Part model, mm, in its own coordinate system. Round coordinates to 2 decimals unless told otherwise and drop trailing zeros. Order: outer loops, then holes, each group sorted by start corner. A loop starts at its lowest first (then second) coordinate and runs counter-clockwise, first axis right, second up. Notation, with made-up numbers: M -8,27.25 L 41,27.25 A30 cw 41,55.25 Z; hole C 77.5,50 d10. An arc over 180 degrees is marked long. One line per question, with ' | ' between items.
from build123d import *

# Parameters (mm, degrees)
TUBE_SQUARE_40_X_40_X_3_2_1_DEPTH = 1920
CUT_EXTRUDE1_DEPTH                = 1921.52076271
SKETCH16_R                        = 2
CUT_EXTRUDE2_DEPTH                = 3
SKETCH17_R                        = 2
CUT_EXTRUDE3_DEPTH                = 3


with BuildPart() as part:
    # Sketch15 → Tube (square) 40 X 40 X 3.2(1) (new body)
    with BuildSketch(Plane(origin=(0, 0, 0), x_dir=(-1, 0, 0), z_dir=(0, 1, 0))):
        with BuildLine():
            Line((-13.6, -20), (13.6, -20))
            ThreePointArc((13.6, -20), (18.1254834, -18.1254834), (20, -13.6))
            Line((20, -13.6), (20, 13.6))
            ThreePointArc((20, 13.6), (18.1254834, 18.1254834), (13.6, 20))
            Line((13.6, 20), (-13.6, 20))
            ThreePointArc((-13.6, 20), (-18.1254834, 18.1254834), (-20, 13.6))
            Line((-20, 13.6), (-20, -13.6))
            ThreePointArc((-20, -13.6), (-18.1254834, -18.1254834), (-13.6, -20))
        make_face()
        with BuildLine():
            Line((-13.6, -16.8), (13.6, -16.8))
            ThreePointArc((13.6, -16.8), (15.8627417, -15.8627417), (16.8, -13.6))
            Line((16.8, -13.6), (16.8, 13.6))
            ThreePointArc((16.8, 13.6), (15.8627417, 15.8627417), (13.6, 16.8))
            Line((13.6, 16.8), (-13.6, 16.8))
            ThreePointArc((-13.6, 16.8), (-15.8627417, 15.8627417), (-16.8, 13.6))
            Line((-16.8, 13.6), (-16.8, -13.6))
            ThreePointArc((-16.8, -13.6), (-15.8627417, -15.8627417), (-13.6, -16.8))
        make_face(mode=Mode.SUBTRACT)
    extrude(amount=TUBE_SQUARE_40_X_40_X_3_2_1_DEPTH)

    # Sketch13 → Cut-Extrude1 (cut, through all)
    with BuildSketch(Plane(origin=(0, 0, -20), x_dir=(-1, 0, 0), z_dir=(0, 0, -1))):
        Polygon((20, 1880), (-20, 1920), (20, 1920), align=None)
    extrude(amount=-CUT_EXTRUDE1_DEPTH, mode=Mode.SUBTRACT)

    # Sketch16 → Cut-Extrude2 (cut)
    with BuildSketch(Plane(origin=(20, 0, 0), x_dir=(0, 0, -1), z_dir=(1, 0, 0))):
        with Locations((0, 1900)):
            Circle(SKETCH16_R)
        with Locations((0, 1447)):
            Circle(SKETCH16_R)
        with Locations((0, 1067)):
            Circle(SKETCH16_R)
        with Locations((0, 687)):
            Circle(SKETCH16_R)
    extrude(amount=-CUT_EXTRUDE2_DEPTH, mode=Mode.SUBTRACT)

    # Sketch17 → Cut-Extrude3 (cut)
    with BuildSketch(Plane.XY.offset(20)):
        with Locations((0, 687)):
            Circle(SKETCH17_R)
    extrude(amount=-CUT_EXTRUDE3_DEPTH, mode=Mode.SUBTRACT)


solid = part.part
1) Probe line 1 (X direction, y = 1227, z = -2); line 2 (Y direction, x = 19.05, z = 0). List the from-to ranges inside material, lowest first. Write a range as [from, to].
The answers:
line 1: x = [-20, -16.8], [16.8, 20] | line 2: y = [0, 685], [689, 1065], [1069, 1445], [1449, 1898], [1902, 1919.05]
2) Drop flat-ended pins along their axis: pin 1 (3.5 mm diameter, centred on y = 1900, z = 0, fed in from -X); pin 2 (1.2 mm diameter, centred on y = 687, z = 1, fed in from +X). Give the stop position or say it passes through.
The answers:
pin 1: stops at x = 16.8 | pin 2: stops at x = 17
3) Saw through at A-A (y = 1798). List the corners of the cut face in (x, z).
The answers:
outline: M -20,-13.6 A6.4 ccw -13.6,-20 L 13.6,-20 A6.4 ccw 20,-13.6 L 20,13.6 A6.4 ccw 13.6,20 L -13.6,20 A6.4 ccw -20,13.6 Z; hole M -16.8,-13.6 A3.2 ccw -13.6,-16.8 L 13.6,-16.8 A3.2 ccw 16.8,-13.6 L 16.8,13.6 A3.2 ccw 13.6,16.8 L -13.6,16.8 A3.2 ccw -16.8,13.6 Z
